from build123d import *

# Parameters (mm, degrees)
SKIZZE1_W                       = 42
SKIZZE1_H                       = 42
SKIZZE1_R                       = 1.7
SKIZZE1_R_2                     = 8.5
AUFSATZ_LINEAR_AUSTRAGEN1_DEPTH = 4
SKIZZE2_R                       = 11.5
SCHNITT_LINEAR_AUSTRAGEN1_DEPTH = 2.4
AUFSATZ_LINEAR_AUSTRAGEN2_DEPTH = 2


with BuildPart() as part:
    # Skizze1 → Aufsatz-Linear austragen1 (new body)
    with BuildSketch(Plane(origin=(0, 0, 0), x_dir=(1, 0, 0), z_dir=(0, 1, 0))):
        Rectangle(SKIZZE1_W, SKIZZE1_H)
        with Locations(Location((-15.5, 15.5, 0), (0, 0, 270))):
            Circle(SKIZZE1_R, mode=Mode.SUBTRACT)
        with Locations(Location((15.5, 15.5, 0), (0, 0, 270))):
            Circle(SKIZZE1_R, mode=Mode.SUBTRACT)
        with Locations(Location((-15.5, -15.5, 0), (0, 0, 270))):
            Circle(SKIZZE1_R, mode=Mode.SUBTRACT)
        with Locations(Location((15.5, -15.5, 0), (0, 0, 270))):
            Circle(SKIZZE1_R, mode=Mode.SUBTRACT)
        with Locations(Location((0, 0, 0), (0, 0, 270))):
            Circle(SKIZZE1_R_2, mode=Mode.SUBTRACT)
    extrude(amount=AUFSATZ_LINEAR_AUSTRAGEN1_DEPTH)

    # Skizze2 → Schnitt-Linear austragen1 (cut)
    with BuildSketch(Plane.XZ):
        with Locations(Location((0, 0, 0), (0, 0, 270))):
            Circle(SKIZZE2_R)
    extrude(amount=-SCHNITT_LINEAR_AUSTRAGEN1_DEPTH, mode=Mode.SUBTRACT)

    # Skizze4 → Aufsatz-Linear austragen2 (add)
    with BuildSketch(Plane.XZ):
        Polygon((-21, -21), (-21, 21), (21, 21), (21, -21), (23, -21), (23, 23), (-23, 23), (-23, -21), align=None)
    extrude(amount=-AUFSATZ_LINEAR_AUSTRAGEN2_DEPTH)


solid = part.part
Could you check a few things on this model? Use its own coordinates, in mm. A direction names the side the tool comes from. Round coordinates to 2 decimals unless told otherwise and drop trailing zeros. Order: outer loops, then holes, each group sorted by start corner. A loop starts at its lowest first (then second) coordinate and runs counter-clockwise, first axis right, second up. Notation, with made-up numbers: M 75,67.5 L 89,67.5 A28 cw 89,93.5 Z; hole C -14.75,13.25 d9. An arc over 180 degrees is marked long. One line per item, written item: value.
(1) Imagine slicing it at A-A (z = -15.5). Write out the boundary of the cut face in (x, y), and give its area (3 significant figures).
Ans:
outline: M -23,0 L -17.2,0 L -17.2,4 L -21,4 L -21,2 L -23,2 Z; M -13.8,0 L 13.8,0 L 13.8,4 L -13.8,4 Z; M 17.2,0 L 23,0 L 23,2 L 21,2 L 21,4 L 17.2,4 Z
area: 149 mm^2
(2) Imagine slicing it at C-C (x = 0). Write out the boundary of the cut face in (y, z).
Ans:
outline: M 0,-21 L 4,-21 L 4,-8.5 L 2.4,-8.5 L 2.4,-11.5 L 0,-11.5 Z; M 0,11.5 L 2.4,11.5 L 2.4,8.5 L 4,8.5 L 4,21 L 2,21 L 2,23 L 0,23 Z
(3) Imagine slicing it at B-B (z = 0). Write out the boundary of the cut face in (x, y), and give its area (3 significant figures).
Ans:
outline: M -23,0 L -11.5,0 L -11.5,2.4 L -8.5,2.4 L -8.5,4 L -21,4 L -21,2 L -23,2 Z; M 8.5,2.4 L 11.5,2.4 L 11.5,0 L 23,0 L 23,2 L 21,2 L 21,4 L 8.5,4 Z
area: 93.6 mm^2
(4) Imagine slicing it at D-D (x = 14.5). Write out the boundary of the cut face in (y, z), and give its area (3 significant figures).
Ans:
outline: M 0,-21 L 4,-21 L 4,-16.87 L 0,-16.87 Z; M 0,-14.13 L 4,-14.13 L 4,14.13 L 0,14.13 Z; M 0,16.87 L 4,16.87 L 4,21 L 2,21 L 2,23 L 0,23 Z
area: 150 mm^2
(5) I'm going to push flat-ended pins straight in: P1, Ø1.6, axis at x = -9.5, y = 3.5, coming from the +Z side; P2, Ø1, axis at y = 3, z = 7.5, coming from the -X side; P3, Ø1, axis at y = 3, z = 3.5, coming from the +X side. Where does each tip first touch, or does it pass through?
Ans:
P1: stops at z = 21
P2: stops at x = -21
P3: stops at x = 21
(6) I need wall thicknesses on line 1 along X through (y, z) = (2.85, 0); line 2 along Z through (x, y) = (19.5, 3.5); line 3 along X through (y, z) = (2.3, -16). Which ranges of each line are inside material? Lowest first, please. Write a range as from..to.
Ans:
line 1: x = -21..-8.5, 8.5..21
line 2: z = -21..21
line 3: x = -21..-17.12, -13.88..13.88, 17.12..21
(7) If we mould it in two halves opening along Z, with no side actions, what happens to faces 1 (the flat face through (-10, 4, 0)), 2 (the flat face through (0, 3, 21)), 3 (the cylindrical face through (-14.99, 1.97, -13.88))? For each: released by +Z, released by -Z, zero draft, split by the parting line, or undercut.
Ans:
face 1: zero draft
face 2: released by +Z
face 3: undercut
(8) Which directions (+Z, -Z, +X, -X, +Y, -Y) give clear straight access to the entire face, cutting with the end or side of a thin tool? Please do faces 4 (the cylindrical face through (9.7, 1.18, -6.18)), 5 (the flat face through (-21, 3, 0)), 6 (the flat face through (0, 2, 22)), 7 (the flat face through (21, 3, 0)).
Ans:
face 4: -Y
face 5: +Z, -Z, -X, +Y
face 6: +Z, +Y
face 7: +Z, -Z, +X, +Y
